Answer from the drawing. Dimensions are ordinates in mm from the lowest x, y and z of the part. A direction names the side the tool comes from. Round coordinates to 2 decimals unless told otherwise and drop trailing zeros. Order: outer loops, then holes, each group sorted by start corner. A loop starts at its lowest first (then second) coordinate and runs counter-clockwise, first axis right, second up. Notation, with made-up numbers: M -26.75,23.5 L 31.25,23.5 A28 ccw 31.25,52.5 Z; hole C -22,27.25 d1. An arc over 180 degrees is marked long. Write item = value, one per line. Start each with the question number.
(1) Straight lines are drawn through the part: probe 1 along Y at (x, z) = (7.5, 7.25); probe 2 along Y at (x, z) = (30, 2.75); probe 3 along Y at (x, z) = (10.5, 8). For each, find the intervals that lie inside material, in ascending order. Write a range as from..to.
(2) For a pull along Y with two mould halves and no side action, classify the marked faces 4, 5 and 6 as released by +Y, released by -Y, zero draft, split by the parting line, or undercut.
(3) A cutting plane is placed at C-C, the plane y = 22.5. Determine the outline of the cut face in (x, z).
(4) A cutting plane is placed at D-D, the plane x = 7.5. Determine the outline of the cut face in (y, z), and give its area (3 significant figures).
(5) A cutting plane is placed at B-B, the plane z = 9. Count the separate pieces of the cut face and the enclosed holes in it, and give its area (3 significant figures).
(6) A cutting plane is placed at A-A, the plane x = 30. Determine the outline of the cut face in (y, z), and give its area (3 significant figures).
(7) Which of the six approach directions +Z, -Z, +X, -X, +Y, -Y give full straight-line access (tool end or side, diameter ignored) to the marked faces 1, 2 and 3?
(8) Each of these flat-tipped pins is pushed along its axis until it touches: pin 1 (4.5 mm diameter, centred on x = 82.5, y = 22.5, fed in from +Z); pin 2 (2 mm diameter, centred on y = 70, z = 4.5, fed in from +X); pin 3 (3 mm diameter, centred on y = 47.5, z = 2.5, fed in from -X); pin 4 (5 mm diameter, centred on x = 80.5, z = 6.5, fed in from +Y). Where does it stop, or does it pass through?
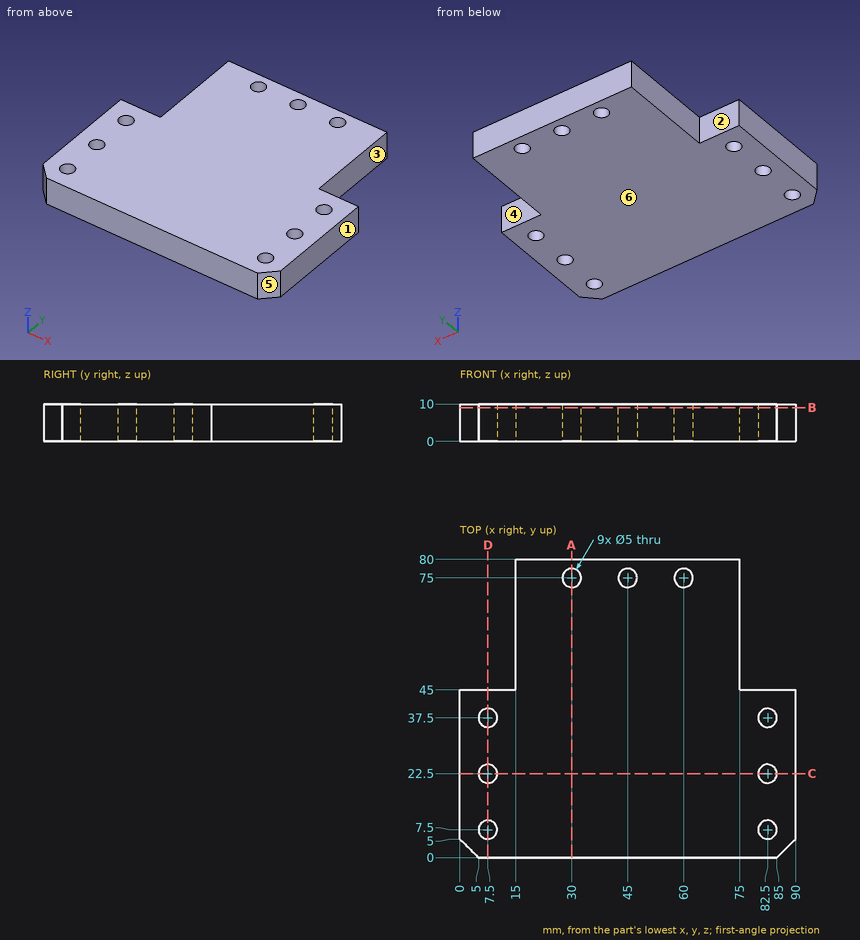
Reported:
q1.probe_1 = 0..5, 10..20, 25..35, 40..45
q1.probe_2 = 0..72.5, 77.5..80
q1.probe_3 = 0..45
q2.face_4 = released by +Y
q2.face_5 = released by -Y
q2.face_6 = zero draft
q3.outline = M 0,0 L 5,0 L 5,10 L 0,10 Z; M 10,0 L 80,0 L 80,10 L 10,10 Z; M 85,0 L 90,0 L 90,10 L 85,10 Z
q4.outline = M 0,0 L 5,0 L 5,10 L 0,10 Z; M 10,0 L 20,0 L 20,10 L 10,10 Z; M 25,0 L 35,0 L 35,10 L 25,10 Z; M 40,0 L 45,0 L 45,10 L 40,10 Z
q4.area = 300 mm²
q5.separate_pieces = 1
q5.enclosed_holes = 9
q5.area = 5,950 mm²
q6.outline = M 0,0 L 72.5,0 L 72.5,10 L 0,10 Z; M 77.5,0 L 80,0 L 80,10 L 77.5,10 Z
q6.area = 750 mm²
q7.face_1 = +Z, -Z, +X, +Y, -Y
q7.face_2 = +Z, -Z, -X, +Y
q7.face_3 = +Z, -Z, +X, +Y
q8.pin_1 = through
q8.pin_2 = 75
q8.pin_3 = 15
q8.pin_4 = 45
